from build123d import *

# Parameters (mm, degrees)
SKETCH2_R   = 9.525
SKETCH2_R_2 = 8.7122


with BuildPart() as part:
    # Sweep1: sweep along a path in Sketch1
    with BuildLine(Plane.XY) as sweep1_path:
        Line((-11.159231637, -185.328818363), (-100.600768363, -95.887281637))
        ThreePointArc((-100.600768363, -95.887281637), (-108.859810189, -83.526752047), (-111.76, -68.946513274))
        Line((-111.76, -68.946513274), (-111.76, 682.844622495))
        ThreePointArc((-111.76, 682.844622495), (-110.461773982, 692.705628113), (-106.655567884, 701.894622495))
        Line((-106.655567884, 701.894622495), (-67.765909488, 769.253486726))
    # Sketch2 → Sweep1 (sweep)
    with BuildSketch(Plane(origin=(0, 0, 0), x_dir=(1, 0, 0), z_dir=(0, 1, 0))):
        with Locations((-111.76, 0)):
            Circle(SKETCH2_R)
        with Locations((-111.76, 0)):
            Circle(SKETCH2_R_2, mode=Mode.SUBTRACT)
    sweep(path=sweep1_path.line)


solid = part.part
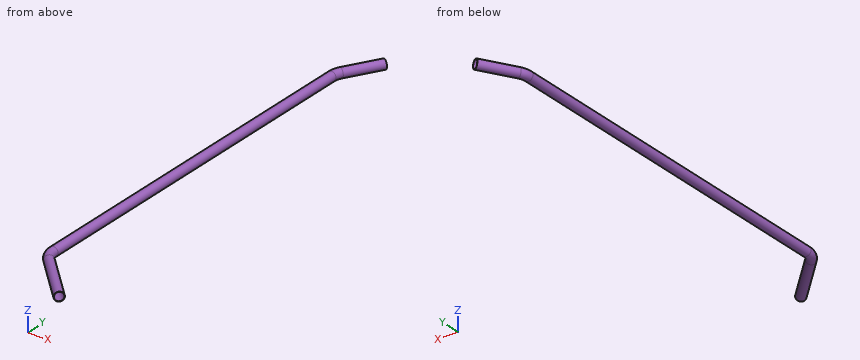
Input: part model. Units: mm. Frame: model coordinates. Round coordinates to 2 decimals unless told otherwise and drop trailing zeros. Order: outer loops, then holes, each group sorted by start corner. A loop starts at its lowest first (then second) coordinate and runs counter-clockwise, first axis right, second up. Notation, with made-up numbers: (66, -21) - (83, -21) arc R21 cw to (83, 11) - close; hole circle Ø11 at (-34, -25.5). An arc over 180 degrees is marked (long way). Answer as a JSON object with one key per item and string values. Group by question number.
(1) Material intervals for probe 1 along Z at (x, y) = (-111.76, 332) (3 decimals); probe 2 along X at (y, z) = (340, 0) (3 decimals); probe 3 along X at (y, z) = (562.5, -1.75), sorted ascending. Write a range as from..to.
(2) Cut plane A-A (z = 3.5). Return loops of the section in (x, y), then the cut area to 3 significant figures.
(3) Cut plane B-B (y = 607.5). Return loops of the section in (x, z) (3 decimals), then the cut area to 3 significant figures.
(4) Pin query (flat end, axial travel): P1, Ø4, axis at y = 645, z = -4, coming from the -X side; P2, Ø8, axis at x = -100.5, z = -3, coming from the +Y side; P3, Ø3, axis at y = 394.5, z = -5, coming from the +X side. Return the tip coordinate at first contact, or that it passes through.
Here are the results:
{
 "1": {"probe 1": "z = -9.525..-8.712, 8.712..9.525", "probe 2": "x = -121.285..-120.472, -103.048..-102.235", "probe 3": "x = -121.12..-120.29, -103.23..-102.4"},
 "2": {"outline": "(-120.62, -68.95) arc R46.96 ccw to (-106.86, -102.15) - (-17.42, -191.59) - (-16.8, -190.97) - (-106.24, -101.53) arc R46.08 cw to (-119.74, -68.95) - (-119.74, 682.84) arc R46.08 cw to (-113.56, 705.88) - (-74.68, 773.24) - (-75.44, 773.68) - (-114.33, 706.32) arc R46.96 ccw to (-120.62, 682.84) - close; (-103.78, -68.95) arc R30.12 ccw to (-94.96, -90.25) - (-5.52, -179.69) - (-4.9, -179.06) - (-94.34, -89.62) arc R29.24 cw to (-102.9, -68.95) - (-102.9, 682.84) arc R29.24 cw to (-98.98, 697.47) - (-60.09, 764.82) - (-60.86, 765.26) - (-99.75, 697.91) arc R30.12 ccw to (-103.78, 682.84) - close", "area": "1,770 mm^2"},
 "3": {"outline": "circle Ø19.05 at (-111.76, 0); hole circle Ø17.424 at (-111.76, 0)", "area": "46.6 mm^2"},
 "4": {"P1": "stops at x = -121.07", "P2": "stops at y = 737.89", "P3": "stops at x = -102.9"}
}
